from build123d import *

# Parameters (mm, degrees)
SKETCH1_W           = 10.5
SKETCH1_H           = 10.5
SKETCH1_W_2         = 4
SKETCH1_H_2         = 10.8
BOSS_EXTRUDE1_DEPTH = 1.65
BOSS_EXTRUDE2_START = 1.65
SKETCH1_3_W         = 4
SKETCH1_3_H         = 10.8
SKETCH1_3_W_2       = 3.06
BOSS_EXTRUDE2_DEPTH = 4.4
BOSS_EXTRUDE3_START = 1.65
SKETCH1_4_W         = 10.5
SKETCH1_4_H         = 10.5
BOSS_EXTRUDE3_DEPTH = 3.86
FILLET1_R           = 1
FILLET2_R           = 1
SKETCH2_W           = 7.790130909
SKETCH2_H           = 1.333210324
CUT_EXTRUDE1_DEPTH  = 2
FILLET3_R           = 1
BOSS_EXTRUDE4_DEPTH = 23.3
FILLET4_R           = 2
FILLET5_R           = 2


with BuildPart() as part:
    # Sketch1 → Boss-Extrude1 (new body)
    with BuildSketch(Plane(origin=(0, 0, 0), x_dir=(1, 0, 0), z_dir=(0, 1, 0))):
        Polygon((17.65, 17.55), (-17.65, 17.55), (-17.65, 0.55), (-13.65, 0.55), (-13.65, -10.25), (-17.65, -10.25), (-17.65, -17.55), (17.65, -17.55), align=None)
        with Locations((-5.88, 7.54)):
            Rectangle(SKETCH1_W, SKETCH1_H, mode=Mode.SUBTRACT)
        with Locations((-15.65, -4.85)):
            Rectangle(SKETCH1_W_2, SKETCH1_H_2)
        with Locations((-5.88, 7.54)):
            Rectangle(SKETCH1_W, SKETCH1_H)
    extrude(amount=BOSS_EXTRUDE1_DEPTH)

    # Sketch1<3> → Boss-Extrude2 (add)
    with BuildSketch(Plane(origin=(0, 0, 0), x_dir=(1, 0, 0), z_dir=(0, 1, 0)).offset(BOSS_EXTRUDE2_START)):
        with Locations((-15.65, -4.85)):
            Rectangle(SKETCH1_3_W, SKETCH1_3_H)
        with Locations((-19.18, -4.85)):
            Rectangle(SKETCH1_3_W_2, SKETCH1_3_H)
    extrude(amount=BOSS_EXTRUDE2_DEPTH)

    # Sketch1<4> → Boss-Extrude3 (add)
    with BuildSketch(Plane(origin=(0, 0, 0), x_dir=(1, 0, 0), z_dir=(0, 1, 0)).offset(BOSS_EXTRUDE3_START)):
        with Locations((-5.88, 7.54)):
            Rectangle(SKETCH1_4_W, SKETCH1_4_H)
    extrude(amount=BOSS_EXTRUDE3_DEPTH)

    # Fillet1
    fillet1_edges = [part.edges().sort_by_distance(p)[0] for p in [
        (-15.65, 1.65, 10.25),
        (-15.65, 1.65, -0.55),
        (-13.65, 1.65, 4.85),
    ]]
    fillet(fillet1_edges, radius=FILLET1_R)

    # Fillet2
    fillet2_edges = [part.edges().sort_by_distance(p)[0] for p in [
        (-17.18, 6.05, -0.55),
        (-20.71, 6.05, 4.85),
        (-17.18, 6.05, 10.25),
        (-13.65, 6.05, 4.85),
    ]]
    fillet(fillet2_edges, radius=FILLET2_R)

    # Sketch2 → Cut-Extrude1 (cut)
    with BuildSketch(Plane.ZY.offset(20.71)):
        with Locations((4.993003368, 3.577240422)):
            Rectangle(SKETCH2_W, SKETCH2_H)
    extrude(amount=-CUT_EXTRUDE1_DEPTH, mode=Mode.SUBTRACT)

    # Fillet3
    fillet3_edges = [part.edges().sort_by_distance(p)[0] for p in [
        (-11.13, 3.58, -2.29),
        (-0.63, 3.58, -2.29),
        (-0.63, 3.58, -12.79),
        (-11.13, 3.58, -12.79),
    ]]
    fillet(fillet3_edges, radius=FILLET3_R)

    # Sketch4 → Boss-Extrude4 (add)
    with BuildSketch(Plane(origin=(17.65, 0, 0), x_dir=(0, 0, -1), z_dir=(1, 0, 0))):
        with BuildLine():
            Line((-5.605, 0), (-5.605, 14.732615083))
            ThreePointArc((-5.605, 14.732615083), (0, 20.337615083), (5.605, 14.732615083))
            Line((5.605, 14.732615083), (5.605, 0))
            Line((5.605, 0), (-5.605, 0))
        make_face()
    extrude(amount=BOSS_EXTRUDE4_DEPTH)

    # Fillet4
    fillet4_edges = [part.edges().sort_by_distance(p)[0] for p in [
        (17.65, 1.65, 0),
    ]]
    fillet(fillet4_edges, radius=FILLET4_R)

    # Fillet5
    fillet5_edges = [part.edges().sort_by_distance(p)[0] for p in [
        (40.95, 0, 0),
    ]]
    fillet(fillet5_edges, radius=FILLET5_R)


solid = part.part
Can you work these out from the model? Positions are in its coordinate system, mm. A direction names the side the tool comes from. Round coordinates to 2 decimals unless told otherwise and drop trailing zeros. Order: outer loops, then holes, each group sorted by start corner. A loop starts at its lowest first (then second) coordinate and runs counter-clockwise, first axis right, second up. Notation, with made-up numbers: M -11,54 L 29,54 A12 ccw 29,61 Z; hole C 15.5,51 d5. An arc over 180 degrees is marked long. Use a Markdown table: item, result.
1) I'm going to push flat-ended pins straight in: P1, Ø3, axis at y = 18, z = -7, coming from the +X side; P2, Ø1.3, axis at y = 1, z = -12.5, coming from the +X side; P3, Ø1, axis at x = -17.5, y = 2.5, coming from the -Z side; P4, Ø1.9, axis at y = 3.5, z = -7, coming from the +X side. Where does each tip first touch, or does it pass through?
Geometry says:
| item | result |
|---|---|
| P1 | passes through |
| P2 | stops at x = 17.65 |
| P3 | stops at z = -0.79 |
| P4 | stops at x = -0.63 |
2) Imagine slicing it at B-B (y = 11.75). List the corners of the cut face in (x, z) for me (3 decimals), then the cut area to 3 significant figures.
Geometry says:
| item | result |
|---|---|
| outline | M 17.65,-5.605 L 40.95,-5.605 L 40.95,5.605 L 17.65,5.605 Z |
| area | 261 mm² |
3) If I drill on line 1 along Y through (x, z) = (-12.5, -8); line 2 along X through (y, z) = (3, 0.5); line 3 along Z through (x, y) = (27, 14.5) (3 decimals), over which ranges is the centre line in solid material (lowest first)?
Geometry says:
| item | result |
|---|---|
| line 1 | y = 0 to 1.65 |
| line 2 | x = -20.71 to -13.65, 17.54 to 40.95 |
| line 3 | z = -5.605 to 5.605 |
4) On a 3-axis mill with a long thin cutter (end or side, diameter ignored), from which of +Z, -Z, +X, -X, +Y, -Y can I reach the whole of each face in a straight line? I mean faces 4 (the face through (-6, 4, -12.79)), 5 (the face through (-17, 4, 10.25)), 6 (the face through (-13.65, 4, 5)). Say none if no direction works.
Geometry says:
| item | result |
|---|---|
| face 4 | -Z, +X, -X, +Y |
| face 5 | +Z, -X, +Y |
| face 6 | +Z, -Z, +Y |
5) If we mould it in two halves opening along Z, with no side actions, what happens to faces 1 (the face through (-20, 4.244, 5)), 2 (the face through (17.65, 1, -11)), 3 (the face through (29.137, 20.336, 0.123))? For each: +Z half, -Z half, draft (parallel to the pull), parting line (faces both ways), or undercut.
Geometry says:
| item | result |
|---|---|
| face 1 | undercut |
| face 2 | draft |
| face 3 | parting line |
6) Imagine slicing it at A-A (x = -16). List the corners of the cut face in (y, z) for me, then the cut area to 3 significant figures.
Geometry says:
| item | result |
|---|---|
| outline | M 0,-17.55 L 1.65,-17.55 L 1.65,-1.55 A1 cw 2.65,-0.55 L 5.05,-0.55 A1 ccw 6.05,0.45 L 6.05,9.25 A1 ccw 5.05,10.25 L 2.65,10.25 A1 cw 1.65,11.25 L 1.65,17.55 L 0,17.55 Z |
| area | 105 mm² |
7) Imagine slicing it at C-C (z = -14). List the corners of the cut face in (x, y) for me, then the cut area to 3 significant figures.
Geometry says:
| item | result |
|---|---|
| outline | M -17.65,0 L 17.65,0 L 17.65,1.65 L -17.65,1.65 Z |
| area | 58.2 mm² |
